Source: CAD feature listing. Evaluate the final solid. Frame: model axes, mm. Give positions to 0.01 mm unless a question says otherwise; leave off trailing zeros. Order: outer loops, then holes, each group sorted by start corner. A loop starts at its lowest first (then second) coordinate and runs counter-clockwise, first axis right, second up.
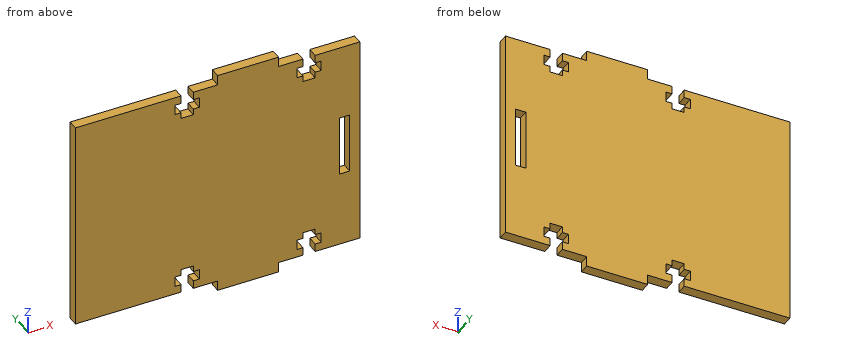
from build123d import *

# Parameters (mm, degrees)
SKETCH1_W           = 3.175
SKETCH1_H           = 19.05
BOSS_EXTRUDE3_DEPTH = 3.175


with BuildPart() as part:
    # Sketch1 → Boss-Extrude3 (new body)
    with BuildSketch(Plane(origin=(0, 0, 0), x_dir=(1, 0, 0), z_dir=(0, 1, 0))):
        Polygon((0, 66.675), (0, 0), (33.02, 0), (33.02, 2.54), (31.115, 2.54), (31.115, 5.715), (33.02, 5.715), (33.02, 7.62), (36.83, 7.62), (36.83, 5.715), (38.735, 5.715), (38.735, 2.54), (36.83, 2.54), (36.83, 0), (44.45, 0), (44.45, -3.175), (63.5, -3.175), (63.5, 0), (71.12, 0), (71.12, 2.54), (69.215, 2.54), (69.215, 5.715), (71.12, 5.715), (71.12, 7.62), (74.93, 7.62), (74.93, 5.715), (76.835, 5.715), (76.835, 2.54), (74.93, 2.54), (74.93, 0), (88.9, 0), (88.9, 66.675), (74.93, 66.675), (74.93, 64.135), (76.835, 64.135), (76.835, 60.96), (74.93, 60.96), (74.93, 59.055), (71.12, 59.055), (71.12, 60.96), (69.215, 60.96), (69.215, 64.135), (71.12, 64.135), (71.12, 66.675), (63.5, 66.675), (63.5, 69.85), (44.45, 69.85), (44.45, 66.675), (36.83, 66.675), (36.83, 64.135), (38.735, 64.135), (38.735, 60.96), (36.83, 60.96), (36.83, 59.055), (33.02, 59.055), (33.02, 60.96), (31.115, 60.96), (31.115, 64.135), (33.02, 64.135), (33.02, 66.675), align=None)
        with Locations((84.1375, 33.3375)):
            Rectangle(SKETCH1_W, SKETCH1_H, mode=Mode.SUBTRACT)
    extrude(amount=BOSS_EXTRUDE3_DEPTH)


solid = part.part
1) Section query B-B on z = -40.5. Output: boundary loops of the cut face in (x, y) (3 decimals), and give its area (3 significant figures).
Checks:
outline: (0, 0) - (82.55, 0) - (82.55, 3.175) - (0, 3.175) - close; (85.725, 0) - (88.9, 0) - (88.9, 3.175) - (85.725, 3.175) - close
area: 272 mm2
2) Section query A-A on z = -3.5. Output: boundary loops of the cut face in (x, y) (3 decimals), and give its area (3 significant figures).
Checks:
outline: (0, 0) - (31.115, 0) - (31.115, 3.175) - (0, 3.175) - close; (38.735, 0) - (69.215, 0) - (69.215, 3.175) - (38.735, 3.175) - close; (76.835, 0) - (88.9, 0) - (88.9, 3.175) - (76.835, 3.175) - close
area: 234 mm2
3) Section query C-C on x = 72.5. Output: boundary loops of the cut face in (y, z) (3 decimals), and give its area (3 significant figures).
Checks:
outline: (0, -59.055) - (3.175, -59.055) - (3.175, -7.62) - (0, -7.62) - close
area: 163 mm2
4) Section query D-D on x = 26.5. Output: boundary loops of the cut face in (y, z) (3 decimals).
Checks:
outline: (0, -66.675) - (3.175, -66.675) - (3.175, 0) - (0, 0) - close
5) Ray query, L1, parallel to Z at x = 37, y = 0.2 (3 decimals); L2, parallel to X at y = 1.6, z = -32.5 (3 decimals); L3, parallel to Z at x = 21.5, y = 1.05 (3 decimals). Return the intervals inside material, ascending.
Checks:
L1: z = -66.675 to -64.135, -60.96 to -5.715, -2.54 to 0
L2: x = 0 to 82.55, 85.725 to 88.9
L3: z = -66.675 to 0
6) First-contact query: pin 1 Ø1 at (x, y) = (72.5, 1.5) entering from -Z (3 decimals); pin 2 Ø1.5 at (x, y) = (70, 2) entering from -Z (3 decimals); pin 3 Ø1.5 at (x, y) = (70, 2) entering from +Z. Flat tips, straight axial feed; report the tip coordinate or a pass-through.
Checks:
pin 1: stops at z = -59.055
pin 2: stops at z = -66.675
pin 3: stops at z = 0
